Geometry check sheet. Reference: drawing and pictorial views, mm from the part's lowest x, y, z. A direction names the side the tool comes from. Coordinates: 2 decimals unless noted, no trailing zeros. Order: outer loops, then holes, each group sorted by start corner. A loop starts at its lowest first (then second) coordinate and runs counter-clockwise, first axis right, second up. Notation, with made-up numbers: M 66.25,13 L 84.25,13 A19 ccw 84.25,36 Z; hole C 81.25,27.5 d2. An arc over 180 degrees is marked long. Return JSON: item names as keys, results as strings.
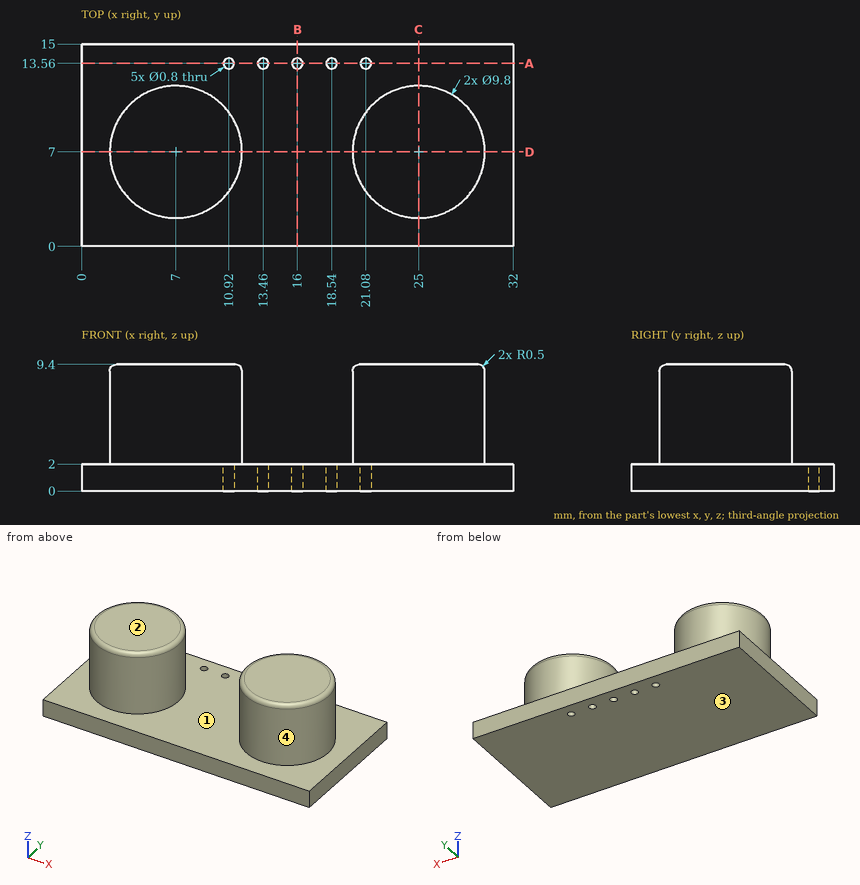
Q1. Cross-section at C-C, the plane x = 25. Record the boundary of the cut face in (y, z).
Values:
{"outline": "M 0,0 L 15,0 L 15,2 L 11.9,2 L 11.9,8.9 A0.5 ccw 11.4,9.4 L 2.6,9.4 A0.5 ccw 2.1,8.9 L 2.1,2 L 0,2 Z"}
Q2. Cross-section at B-B, the plane x = 16. Record the boundary of the cut face in (y, z), and give its area (3 significant figures).
Values:
{"outline": "M 0,0 L 13.16,0 L 13.16,2 L 0,2 Z; M 13.96,0 L 15,0 L 15,2 L 13.96,2 Z", "area": "28.4 mm^2"}
Q3. Material ranges on line 1 along X through (y, z) = (13.56, 0.5); line 2 along Y through (x, z) = (10.92, 1.4); line 3 along Z through (x, y) = (9, 2.25), recorded low to high.
Values:
{"line 1": "0 to 10.52, 11.32 to 13.06, 13.86 to 15.6, 16.4 to 18.14, 18.94 to 20.68, 21.48 to 32", "line 2": "0 to 13.16, 13.96 to 15", "line 3": "0 to 2"}
Q4. Draft check along X on the marked faces 1 and 2. Enter one of: pulls with the +X half, pulls with the -X half, needs draft (parallel to the pull), parting line crosses it, or undercut.
Values:
{"face 1": "undercut", "face 2": "needs draft"}
Q5. Go/stop test with flat-tipped pins: pin 1 (4 mm diameter, centred on x = 5.5, z = 6, fed in from -Y); pin 2 (1 mm diameter, centred on y = 9, z = 6.5, fed in from +X). Record where each tip stops, or that it passes through.
Values:
{"pin 1": "y = 2.1", "pin 2": "x = 29.66"}
Q6. Tool access check on the marked faces 3 and 4. Record the directions out of +Z, -Z, +X, -X, +Y, -Y that give a thin tool (end or side, any length) a straight path to the whole face; none if there is none.
Values:
{"face 3": "-Z, +X, -X, +Y, -Y", "face 4": "+Z"}
Q7. Cross-section at D-D, the plane y = 7. Record the boundary of the cut face in (x, z).
Values:
{"outline": "M 0,0 L 32,0 L 32,2 L 29.9,2 L 29.9,8.9 A0.5 ccw 29.4,9.4 L 20.6,9.4 A0.5 ccw 20.1,8.9 L 20.1,2 L 11.9,2 L 11.9,8.9 A0.5 ccw 11.4,9.4 L 2.6,9.4 A0.5 ccw 2.1,8.9 L 2.1,2 L 0,2 Z"}
Q8. Cross-section at A-A, the plane y = 13.56. Record the boundary of the cut face in (x, z).
Values:
{"outline": "M 0,0 L 10.52,0 L 10.52,2 L 0,2 Z; M 11.32,0 L 13.06,0 L 13.06,2 L 11.32,2 Z; M 13.86,0 L 15.6,0 L 15.6,2 L 13.86,2 Z; M 16.4,0 L 18.14,0 L 18.14,2 L 16.4,2 Z; M 18.94,0 L 20.68,0 L 20.68,2 L 18.94,2 Z; M 21.48,0 L 32,0 L 32,2 L 21.48,2 Z"}
